Input: part model. Units: mm. Frame: model coordinates. Coordinates: 2 decimals unless noted, no trailing zeros. Write each loop counter-clockwise with the first axis right and the second up, starting at its lowest first coordinate (ties: lowest second). Pieces come first, ordered by that corner, then holes. Notation, with made-up numbers: (83, 7.5) - (104, 7.5) arc R33 ccw to (104, 41.5) - close; hole circle Ø5 at (73.25, 15.25). An arc over 180 degrees is marked (long way). One line per question, with ' | ' between items. Start each with the question number.
1) First-contact query: P1, Ø4, axis at x = 401, z = -34, coming from the +Y side. Flat tip, straight axial feed; report the tip coordinate or a pass-through.
2) Line query: line 1 (Z direction, x = 519.5, y = 0.5); line 2 (Z direction, x = 159, y = 0.6); line 3 (X direction, y = 1.05, z = -155). Output: solid intervals per line, ascending.
3) Section query B-B on z = -155. Return loops of the section in (x, y), and give its area (3 significant figures).
4) Section query A-A on x = 41. Return loops of the section in (y, z).
5) Draft query along Z for faces 1 (the cylindrical face through (526.436, 1.521, -34.976)), 2 (the flat face through (276, 0, -157)). Return one class per face: released by +Z, released by -Z, zero draft, split by the parting line, or undercut.
```python
from build123d import *

# Parameters (mm, degrees)
SKETCH2_W           = 560
SKETCH2_H           = 310
BOSS_EXTRUDE1_DEPTH = 3
SKETCH3_R           = 2.15
CUT_EXTRUDE1_DEPTH  = 641.085150585
SKETCH4_R           = 5.15
CUT_EXTRUDE2_DEPTH  = 641.085150585
SKETCH5_R           = 7.5
CUT_EXTRUDE3_DEPTH  = 641.085150585


with BuildPart() as part:
    # Sketch2 → Boss-Extrude1 (new body)
    with BuildSketch(Plane(origin=(0, 0, 0), x_dir=(1, 0, 0), z_dir=(0, 1, 0))):
        with Locations((280, 155)):
            Rectangle(SKETCH2_W, SKETCH2_H)
    extrude(amount=BOSS_EXTRUDE1_DEPTH)

    # Sketch3 → Cut-Extrude1 (cut, through all)
    with BuildSketch(Plane(origin=(0, 3, 0), x_dir=(1, 0, 0), z_dir=(0, 1, 0))):
        with Locations(Location((159, 276, 0), (0, 0, 270))):
            Circle(SKETCH3_R)
        with Locations(Location((401, 276, 0), (0, 0, 270))):
            Circle(SKETCH3_R)
        with Locations(Location((401, 34, 0), (0, 0, 270))):
            Circle(SKETCH3_R)
        with Locations(Location((159, 34, 0), (0, 0, 270))):
            Circle(SKETCH3_R)
    extrude(amount=-CUT_EXTRUDE1_DEPTH, mode=Mode.SUBTRACT)

    # Sketch4 → Cut-Extrude2 (cut, through all)
    with BuildSketch(Plane(origin=(0, 3, 0), x_dir=(1, 0, 0), z_dir=(0, 1, 0))):
        with Locations(Location((41, 155, 0), (0, 0, 270))):
            Circle(SKETCH4_R)
        with Locations(Location((519, 155, 0), (0, 0, 270))):
            Circle(SKETCH4_R)
    extrude(amount=-CUT_EXTRUDE2_DEPTH, mode=Mode.SUBTRACT)

    # Sketch5 → Cut-Extrude3 (cut, through all)
    with BuildSketch(Plane(origin=(0, 3, 0), x_dir=(1, 0, 0), z_dir=(0, 1, 0))):
        with Locations(Location((41, 34, 0), (0, 0, 270))):
            Circle(SKETCH5_R)
        with Locations(Location((41, 276, 0), (0, 0, 270))):
            Circle(SKETCH5_R)
        with Locations(Location((519, 276, 0), (0, 0, 270))):
            Circle(SKETCH5_R)
        with Locations(Location((519, 34, 0), (0, 0, 270))):
            Circle(SKETCH5_R)
    extrude(amount=-CUT_EXTRUDE3_DEPTH, mode=Mode.SUBTRACT)


solid = part.part
```
Answer key:
1) P1: through
2) line 1: -310 to -283.48, -268.52 to -160.13, -149.87 to -41.48, -26.52 to 0 | line 2: -310 to -278.15, -273.85 to -36.15, -31.85 to 0 | line 3: 0 to 35.85, 46.15 to 513.85, 524.15 to 560
3) outline: (0, 0) - (35.85, 0) - (35.85, 3) - (0, 3) - close; (46.15, 0) - (513.85, 0) - (513.85, 3) - (46.15, 3) - close; (524.15, 0) - (560, 0) - (560, 3) - (524.15, 3) - close | area: 1,620 mm²
4) outline: (0, -310) - (3, -310) - (3, -283.5) - (0, -283.5) - close; (0, -268.5) - (3, -268.5) - (3, -160.15) - (0, -160.15) - close; (0, -149.85) - (3, -149.85) - (3, -41.5) - (0, -41.5) - close; (0, -26.5) - (3, -26.5) - (3, 0) - (0, 0) - close
5) face 1: undercut | face 2: zero draft
